```python
from build123d import *

# Parameters (mm, degrees)
F0_W      = 50.8
F0_H      = 50.8
F0_R      = 3.4925
F1_DEPTH  = 38.1
F2_W      = 17.272
F2_H      = 27.94
F3_DEPTH  = 43.18
F4_R      = 5.08
F5_DEPTH  = 36.449
F6_DEPTH  = 2.54
F7_DEPTH  = 31.75
F9_W      = 31.1426110566
F9_H      = 46.6452091932
F10_DEPTH = 31.75
F8_R      = 10.4775
F11_DEPTH = 25.4
F12_R     = 11.43
F13_DEPTH = 7.4676
F14_DEPTH = 10.16
F15_DEPTH = 10.16
F16_R     = 18.3963073453
F17_R     = 3.175
F18_DEPTH = 57.912


with BuildPart() as f1:
    # F0 (on Front) → F1 (new body)
    with BuildSketch(Plane.XZ):
        Rectangle(F0_W, F0_H)
        with Locations((-12.7, -12.7)):
            Circle(F0_R, mode=Mode.SUBTRACT)
        with Locations((12.7, -12.7)):
            Circle(F0_R, mode=Mode.SUBTRACT)
        with Locations((-12.7, 12.7)):
            Circle(F0_R, mode=Mode.SUBTRACT)
        with Locations((12.7, 12.7)):
            Circle(F0_R, mode=Mode.SUBTRACT)
    extrude(amount=F1_DEPTH)

    # F2 (on face) → F3 (cut)
    with BuildSketch(Plane.XY.offset(25.4)):
        with Locations((14.8867284879, -22.0405142754)):
            Rectangle(F2_W, F2_H)
        with Locations((-14.7609785199, -22.0405142754)):
            Rectangle(F2_W, F2_H)
    extrude(amount=-F3_DEPTH, mode=Mode.SUBTRACT)

    # F4 (on face) → F5 (cut)
    with BuildSketch(Plane.XZ.offset(38.1)):
        with Locations((-12.7, 12.7)):
            Circle(F4_R)
        with Locations((12.7, 12.7)):
            Circle(F4_R)
        with Locations((-12.7, -12.7)):
            Circle(F4_R)
        with Locations((12.7, -12.7)):
            Circle(F4_R)
    extrude(amount=-F5_DEPTH, mode=Mode.SUBTRACT)

    # F6 (add): a face of the model
    f6_faces = [f1.faces().sort_by_distance(p)[0] for p in [
        (0, 0, 0),
    ]]
    extrude(f6_faces, amount=F6_DEPTH)

    # F7 (add): a face of the model
    f7_faces = [f1.faces().sort_by_distance(p)[0] for p in [
        (25.4, -17.78, 0),
    ]]
    extrude(f7_faces, amount=F7_DEPTH)

    # F9 (on face) → F10 (cut)
    with BuildSketch(Plane(origin=(0, 2.54, 0), x_dir=(-1, 0, 0), z_dir=(0, 1, 0))):
        with Locations((-39.3411628902, 0)):
            Rectangle(F9_W, F9_H)
    extrude(amount=-F10_DEPTH, mode=Mode.SUBTRACT)

    # F8 (on face) → F11 (cut)
    with BuildSketch(Plane.XZ.offset(38.1)):
        with Locations((41.275, 0)):
            Circle(F8_R)
    extrude(amount=-F11_DEPTH, mode=Mode.SUBTRACT)

    # F12 (on face) → F13 (cut)
    with BuildSketch(Plane(origin=(0, -29.21, 0), x_dir=(-1, 0, 0), z_dir=(0, 1, 0))):
        with Locations((-41.275, 0)):
            Circle(F12_R)
    extrude(amount=-F13_DEPTH, mode=Mode.SUBTRACT)

    # F14 (add): a face of the model
    f14_faces = [f1.faces().sort_by_distance(p)[0] for p in [
        (39.3411628902, -13.335, 23.3226045966),
    ]]
    extrude(f14_faces, amount=F14_DEPTH)

    # F15 (add): a face of the model
    f15_faces = [f1.faces().sort_by_distance(p)[0] for p in [
        (39.3411628902, -13.335, -23.3226045966),
    ]]
    extrude(f15_faces, amount=F15_DEPTH)

    # F16
    f16_edges = [f1.edges().sort_by_distance(p)[0] for p in [
        (57.15, -17.78, 25.4),
        (57.15, -17.78, -25.4),
    ]]
    fillet(f16_edges, radius=F16_R)

    # F17 (on face) → F18 (cut, symmetric)
    with BuildSketch(Plane(origin=(0, 0, 13.1626045966), x_dir=(1, 0, 0), z_dir=(0, 0, -1))):
        with Locations((30.2186440676, 2.5074067526)):
            Circle(F17_R)
    extrude(amount=F18_DEPTH, both=True, mode=Mode.SUBTRACT)


solid = f1.part
```
The model under review builds one solid part; all positions refer to its coordinate system, in mm. A direction names the side the tool comes from. Coordinates: 2 decimals unless noted, no trailing zeros. Write each loop counter-clockwise with the first axis right and the second up, starting at its lowest first coordinate (ties: lowest second). Pieces come first, ordered by that corner, then holes.
1) Machinability: for faces 1 (the face through (11.6, -37.07, -17.66)), 2 (the face through (40, -13, 13.163)), 3 (the face through (15, -22, -17.78)), which of the approach directions +Z, -Z, +X, -X, +Y, -Y give a long, thin tool a straight path to every point of the face, cutting with its end or side? Answer none if there is none.
2) We need section A-A on z = 0. Count the separate pieces of the cut face and the enclosed holes in it, then the cut area to 3 significant figures.
3) The part is to be moulded in two halves that separate along Y. For faces 4 (the face through (-13.361, -4.906, 17.737)), 5 (the face through (15, -36.011, 4)), 6 (the face through (-6.125, -22, 4)), 7 (the face through (-9, -1.651, -11)), say which applies: pulls with the +Y half, pulls with the -Y half, needs draft (parallel to the pull), parting line crosses it, or undercut.
4) Clearance check with flat-ended pins moving along their axes: pin 1 Ø5 at (x, z) = (-14.5, 14.5) entering from -Y; pin 2 Ø8 at (x, z) = (-11.5, -12) entering from -Y; pin 3 Ø2 at (x, y) = (-11.5, -19.5) entering from +Z. State where each tip first meets the part, or that it passes through.
5) To check wall thickness, follow probe 1 along X at (y, z) = (-23.5, 6); probe 2 along Z at (x, y) = (-12.7, -36.65); probe 3 along Y at (x, z) = (-18, 21). State the ranges of each line that lie inside material, in increasing order.
6) We need section C-C on z = -6. State the section outline as (x, y) points, then the cut area to 3 significant figures.
7) We need section B-B on y = -21. State the section outline as (x, z) points.
Answer list:
1. face 1: -Y
1. face 2: +Y
1. face 3: +Z
2. separate pieces: 2
2. enclosed holes: 2
2. area: 1,200 mm2
3. face 4: needs draft
3. face 5: undercut
3. face 6: undercut
3. face 7: pulls with the -Y half
4. pin 1: stops at y = -1.65
4. pin 2: stops at y = -38.1
4. pin 3: stops at z = -17.78
5. probe 1: x = -25.4 to -23.4, -6.12 to 6.25, 23.52 to 23.77, 54.91 to 57.15
5. probe 2: z = -25.4 to -17.78, -7.62 to 7.62, 17.78 to 25.4
5. probe 3: y = -38.1 to -36.01, -8.07 to 2.54
6. outline: (-25.4, -38.1) - (32.69, -38.1) - (32.69, -36.68) - (31.55, -36.68) - (31.55, -29.21) - (23.77, -29.21) - (23.77, 2.54) - (-25.4, 2.54) - close; (49.86, -38.1) - (57.15, -38.1) - (57.15, 2.54) - (54.91, 2.54) - (54.91, -29.21) - (51, -29.21) - (51, -36.68) - (49.86, -36.68) - close; hole (-23.4, -36.01) - (-6.12, -36.01) - (-6.12, -8.07) - (-23.4, -8.07) - close; hole (6.25, -36.01) - (23.52, -36.01) - (23.52, -8.07) - (6.25, -8.07) - close
6. area: 1,230 mm2
7. outline: (-25.4, -25.4) - (38.75, -25.4) arc R18.4 ccw to (57.15, -7) - (57.15, 7) arc R18.4 ccw to (38.75, 25.4) - (23.52, 25.4) - (23.52, -17.78) - (6.25, -17.78) - (6.25, 25.4) - (-6.12, 25.4) - (-6.12, -17.78) - (-23.4, -17.78) - (-23.4, 25.4) - (-25.4, 25.4) - close; hole (23.77, -13.16) - (54.91, -13.16) - (54.91, 13.16) - (23.77, 13.16) - close
